CAD build for the part. Positions are in the model's coordinates, mm. A direction names the side the tool comes from. Coordinates: 2 decimals unless noted, no trailing zeros. Order: outer loops, then holes, each group sorted by start corner. A loop starts at its lowest first (then second) coordinate and runs counter-clockwise, first axis right, second up. Notation, with made-up numbers: (-15.5, 23.25) - (1.5, 23.25) arc R10 ccw to (1.5, 34.25) - close; hole circle Ø10 at (73.25, 31.25). An arc over 180 degrees is marked (long way). Write each question's results on one line, items separated by ' | '. Start each with the question number.
Q1. Pin check, flat tips, straight feed: P1, Ø2, axis at x = -3.5, z = 2.5, coming from the +Y side; P2, Ø3, axis at x = -9.5, y = 2.5, coming from the +Z side; P3, Ø2, axis at x = -8, y = 2.5, coming from the +Z side; P4, Ø2.5, axis at x = -0.5, z = 0.5, coming from the -Y side. Stop position of each tip, or through.
Q2. Wall check: probe 1 along Y at (x, z) = (5.25, -1); probe 2 along Z at (x, y) = (0, 1.45); probe 3 along Z at (x, y) = (-8.5, 4.75). Give the ranges that are in metal, low to high.
Q3. Band-saw the part on B-B, the plane y = 2.5. Write the cut outline in (x, z), then the cut area to 3 significant figures.
Q4. Which spindle directions (+Z, -Z, +X, -X, +Y, -Y) get a long thin tool onto all of the face, cutting with end or side? Do faces 1 (the flat face through (-6.423, -0.5, -3.5)), 2 (the flat face through (5.4, 5.5, -2.5)), 3 (the flat face through (0, 6, -1)), 4 (the flat face through (-6.423, 5.5, 0)). Say none if no direction does.
Q5. Band-saw the part on D-D, the plane z = -3.25. Write the cut outline in (x, y).
Q6. Band-saw the part on A-A, the plane z = 0. Write the cut outline in (x, y), then the cut area to 3 significant figures.
Q7. Pull direction Z, two halves, no side cores. Call faces 5 (the flat face through (-12, 3, 1)), 6 (the flat face through (0, 8, -3)), 7 (the cylindrical face through (4.2, 2.46, 1.61)): released by +Z, released by -Z, zero draft, split by the parting line, or undercut.
Q8. Band-saw the part on C-C, the plane x = -10. Write the cut outline in (y, z), then the cut area to 3 significant figures.
```python
from build123d import *

# Parameters (mm, degrees)
BOSS_EXTRUDE1_DEPTH = 5
BOSS_EXTRUDE2_REACH = 17.411
SKETCH3_W           = 6.077383711
SKETCH3_H           = 1
SKETCH4_W           = 1.5
SKETCH4_H           = 7
CUT_EXTRUDE1_DEPTH  = 10
SKETCH2_R           = 2
CUT_EXTRUDE2_DEPTH  = 10
BOSS_EXTRUDE3_DEPTH = 1
BOSS_EXTRUDE4_DEPTH = 2
SKETCH7_R           = 1.75
BOSS_EXTRUDE5_DEPTH = 13
FILLET1_R           = 1


with BuildPart() as part:
    # Sketch1 → Boss-Extrude1 (new body)
    with BuildSketch(Plane(origin=(0, 0, 0), x_dir=(1, 0, 0), z_dir=(0, 1, 0))):
        with BuildLine():
            Line((-4.69041576, 4.5), (-12.5, 4.5))
            Line((-12.5, 4.5), (-12.5, 2.5))
            Line((-12.5, 2.5), (-3.741657387, 2.5))
            ThreePointArc((-3.741657387, 2.5), (4.133186129, -1.779542756), (-4.387482194, 1))
            Line((-4.387482194, 1), (-12.5, 1))
            Line((-12.5, 1), (-12.5, -1))
            Line((-12.5, -1), (-6.422616289, -1))
            ThreePointArc((-6.422616289, -1), (6.199787926, -1.952595623), (-4.69041576, 4.5))
        make_face()
    extrude(amount=BOSS_EXTRUDE1_DEPTH)

    # Boss-Extrude2: up to this face of the body (flat: up to its plane)
    boss_extrude2_end = Plane(part.part.faces().sort_by_distance((-8.59520788, 2.5, -4.5))[0])
    # Sketch3 → Boss-Extrude2 (add, up to the picked face)
    with BuildSketch(Plane.XY.offset(1), mode=Mode.PRIVATE) as boss_extrude2_sk1:
        with Locations((-9.461308145, 5.5)):
            Rectangle(SKETCH3_W, SKETCH3_H)
    boss_extrude2_tool1 = split(extrude(boss_extrude2_sk1.sketch, amount=-BOSS_EXTRUDE2_REACH, mode=Mode.PRIVATE), bisect_by=boss_extrude2_end, keep=Keep.BOTH, mode=Mode.PRIVATE)
    # Sketch3 → Boss-Extrude2 (add, up to the picked face)
    with BuildSketch(Plane.XY.offset(1), mode=Mode.PRIVATE) as boss_extrude2_sk2:
        with Locations((-9.461308145, -0.5)):
            Rectangle(SKETCH3_W, SKETCH3_H)
    boss_extrude2_tool2 = split(extrude(boss_extrude2_sk2.sketch, amount=-BOSS_EXTRUDE2_REACH, mode=Mode.PRIVATE), bisect_by=boss_extrude2_end, keep=Keep.BOTH, mode=Mode.PRIVATE)
    add(boss_extrude2_tool1.solids().sort_by(Axis((-9.461308, 5.5, 1), (0, 0, -1)))[0])
    add(boss_extrude2_tool2.solids().sort_by(Axis((-9.461308, -0.5, 1), (0, 0, -1)))[0])

    # Sketch4 → Cut-Extrude1 (cut)
    with BuildSketch(Plane.ZY.offset(12.5)):
        with Locations((-1.75, 2.5)):
            Rectangle(SKETCH4_W, SKETCH4_H)
    extrude(amount=-CUT_EXTRUDE1_DEPTH, mode=Mode.SUBTRACT)

    # Sketch2 → Cut-Extrude2 (cut)
    with BuildSketch(Plane.XY.offset(1)):
        with Locations((-9.461308145, 2.5)):
            Circle(SKETCH2_R)
    extrude(amount=-CUT_EXTRUDE2_DEPTH, mode=Mode.SUBTRACT)

    # Sketch5 → Boss-Extrude3 (add)
    with BuildSketch(Plane(origin=(0, 5, 0), x_dir=(1, 0, 0), z_dir=(0, 1, 0))):
        with BuildLine():
            Line((4.898979486, 2.5), (6, 2.5))
            ThreePointArc((6, 2.5), (0, 6.5), (-6, 2.5))
            Line((-6, 2.5), (-4.898979486, 2.5))
            ThreePointArc((-4.898979486, 2.5), (0, 5.5), (4.898979486, 2.5))
        make_face()
    extrude(amount=BOSS_EXTRUDE3_DEPTH)

    # Sketch6 → Boss-Extrude4 (add)
    with BuildSketch(Plane(origin=(0, 6, 0), x_dir=(1, 0, 0), z_dir=(0, 1, 0))):
        with BuildLine():
            Line((-6.048440472, -2.380413381), (6.048440472, -2.380413381))
            ThreePointArc((6.048440472, -2.380413381), (0, 6.5), (-6.048440472, -2.380413381))
        make_face()
    extrude(amount=BOSS_EXTRUDE4_DEPTH)

    # Sketch7 → Boss-Extrude5 (add)
    with BuildSketch(Plane(origin=(0, 8, 0), x_dir=(1, 0, 0), z_dir=(0, 1, 0))):
        with Locations(Location((0, 0, 0), (0, 0, 90))):
            Circle(SKETCH7_R)
    extrude(amount=BOSS_EXTRUDE5_DEPTH)

    # Fillet1
    fillet1_edges = [part.edges().sort_by_distance(p)[0] for p in [
        (0, 8, 1.75),
    ]]
    fillet(fillet1_edges, radius=FILLET1_R)


solid = part.part
```
Results below:
1) P1: stops at y = 8 | P2: passes through | P3: stops at z = 1 | P4: stops at y = 6
2) probe 1: y = 0 to 5, 6 to 8 | probe 2: z = -6.5 to -4.5, 4.5 to 6.5 | probe 3: z = -4.5 to -2.5, -1 to 1
3) outline: (-12.5, -4.5) - (-11.46, -4.5) - (-11.46, -2.5) - (-12.5, -2.5) - close; (-12.5, -1) - (-11.46, -1) - (-11.46, 1) - (-12.5, 1) - close; (-7.46, -4.5) - (-4.69, -4.5) arc R6.5 ccw (long way) to (-6.42, 1) - (-7.46, 1) - (-7.46, -1) - (-4.39, -1) arc R4.5 cw (long way) to (-3.74, -2.5) - (-7.46, -2.5) - close | area: 76.1 mm²
4) face 1: +Z, -Z, +X, -Y | face 2: +Z, +X, -X | face 3: +Z | face 4: +Z, -Z, +X
5) outline: (-12.5, -1) - (-6.42, -1) - (-6.42, 0) - (-3.11, 0) - (-3.11, 5) - (-4.44, 5) - (-4.44, 6) - (4.44, 6) - (4.44, 5) - (3.11, 5) - (3.11, 0) - (5.63, 0) - (5.63, 8) - (-5.63, 8) - (-5.63, 5) - (-6.42, 5) - (-6.42, 6) - (-12.5, 6) - close; hole circle Ø4 at (-9.46, 2.5)
6) outline: (-12.5, -1) - (-6.42, -1) - (-6.42, 0) - (-4.5, 0) - (-4.5, 5) - (-6.42, 5) - (-6.42, 6) - (6.5, 6) - (6.5, 8) - (2.75, 8) arc R1 cw to (1.75, 9) - (1.75, 21) - (-1.75, 21) - (-1.75, 9) arc R1 cw to (-2.75, 8) - (-6.5, 8) - (-6.5, 6) - (-12.5, 6) - close; (4.5, 0) - (6.5, 0) - (6.5, 5) - (4.5, 5) - close; hole circle Ø4 at (-9.46, 2.5) | area: 122 mm²
7) face 5: released by +Z | face 6: zero draft | face 7: undercut
8) outline: (-1, -4.5) - (0.57, -4.5) - (0.57, -2.5) - (-1, -2.5) - close; (-1, -1) - (0.57, -1) - (0.57, 1) - (-1, 1) - close; (4.43, -4.5) - (6, -4.5) - (6, -2.5) - (4.43, -2.5) - close; (4.43, -1) - (6, -1) - (6, 1) - (4.43, 1) - close | area: 12.6 mm²
